```python
from build123d import *

# Parameters (mm, degrees)
F0_R     = 20
F0_R_2   = 2.25
F1_DEPTH = 22
F2_R     = 20
F2_R_2   = 14.25
F3_DEPTH = 7
F5_DEPTH = 13


with BuildPart() as f1:
    # F0 (on Right) → F1 (new body)
    with BuildSketch(Plane.YZ):
        Circle(F0_R)
        with Locations((-9.526279, -5.5)):
            Circle(F0_R_2, mode=Mode.SUBTRACT)
        with Locations((9.526279, -5.5)):
            Circle(F0_R_2, mode=Mode.SUBTRACT)
        with Locations((0, 11)):
            Circle(F0_R_2, mode=Mode.SUBTRACT)
    extrude(amount=F1_DEPTH)

    # F2 (on face) → F3 (join)
    with BuildSketch(Plane(origin=(0, 0, 0), x_dir=(0, -1, 0), z_dir=(-1, 0, 0))):
        Circle(F2_R)
        Circle(F2_R_2, mode=Mode.SUBTRACT)
    extrude(amount=F3_DEPTH)

    # F4 (on face) → F5 (cut)
    with BuildSketch(Plane.YZ.offset(22)):
        Polygon((3.752777, 6.5), (-3.752777, 6.5), (-7.505553, 0), (-3.752777, -6.5), (3.752777, -6.5), (7.505553, 0), align=None)
    extrude(amount=-F5_DEPTH, mode=Mode.SUBTRACT)


solid = f1.part
```
Input: part model. Units: mm. Frame: model coordinates. A direction names the side the tool comes from. Round coordinates to 2 decimals unless told otherwise and drop trailing zeros. Loops run counter-clockwise (first coordinate to the right, second up) from the corner with the lowest first, then second, coordinate; pieces in that order, holes last. Notation, with made-up numbers: M 8,-36.5 L 39,-36.5 A22 cw 39,-2.5 Z; hole C 27,3.5 d7. An arc over 180 degrees is marked long. Answer in a Markdown table with one row per item. Add a question column.
1. Section C-C (x = 5). Output: boundary loops of the cut face in (y, z), and give its area (3 significant figures).
2. Set-up query: faces 1 (the face through (-3.451, -13.163, -5.458)), 2 (the face through (10.85, -0.29, 13.23)), 3 (the face through (16, 0, 6.5)). Return all of +Z, -Z, +X, -X, +Y, -Y with unobstructed straight access to the full face (end or side cutting, diameter ignored); none if empty.
3. Contact query for flat-ended pins moving along their axis: pin 1 (4 mm diameter, centred on y = -9.53, z = -5.5, fed in from -X); pin 2 (10 mm diameter, centred on x = 16.5, z = -7.5, fed in from -Y); pin 3 (1 mm diameter, centred on x = 5.5, y = -5, fed in from -Z); pin 4 (4 mm diameter, centred on x = 17.5, y = -1.5, fed in from +Z). Output: stop coordinate, or through.
4. Section D-D (z = -9.5). Output: boundary loops of the cut face in (x, y).
5. Mould query, pull axis Z, two halves, no side actions, for faces 4 (the face through (10.85, -7.38, -4.82)), 5 (the face through (-7, 5, 14)), 6 (the face through (15.59, -5.66, -3.2)). Classes: released by +Z, released by -Z, zero draft, split by the parting line, or undercut.
6. Section B-B (z = 11). Output: boundary loops of the cut face in (x, y).
7. Section A-A (y = 0). Output: boundary loops of the cut face in (x, z), and give its area (4 significant figures).
8. Ray query, probe 1 along Z at (x, y) = (17, 0); probe 2 along Y at (x, z) = (18.25, -7) (3 decimals); probe 3 along Y at (x, z) = (12.5, 0). Return the intervals inside material, ascending.
Values follow:
| question | item | result |
|---|---|---|
| 1 | outline | C 0,0 d40; hole C -9.53,-5.5 d4.5; hole C 0,11 d4.5; hole C 9.53,-5.5 d4.5 |
| 1 | area | 1,210 mm^2 |
| 2 | face 1 | -X |
| 2 | face 2 | +X, -X |
| 2 | face 3 | +X |
| 3 | pin 1 | through |
| 3 | pin 2 | y = -19.84 |
| 3 | pin 3 | z = -19.49 |
| 3 | pin 4 | z = 20 |
| 4 | outline | M -7,-17.6 L 22,-17.6 L 22,17.6 L -7,17.6 L -7,10.62 L 0,10.62 L 0,-10.62 L -7,-10.62 Z |
| 5 | face 4 | undercut |
| 5 | face 5 | zero draft |
| 5 | face 6 | undercut |
| 6 | outline | M -7,-16.7 L 22,-16.7 L 22,-2.25 L 0,-2.25 L 0,-9.06 L -7,-9.06 Z; M -7,9.06 L 0,9.06 L 0,2.25 L 22,2.25 L 22,16.7 L -7,16.7 Z |
| 7 | outline | M -7,-20 L 22,-20 L 22,-6.5 L 9,-6.5 L 9,6.5 L 22,6.5 L 22,8.75 L 0,8.75 L 0,-14.25 L -7,-14.25 Z; M -7,14.25 L 0,14.25 L 0,13.25 L 22,13.25 L 22,20 L -7,20 Z |
| 7 | area | 692.5 mm^2 |
| 8 | probe 1 | -20 to -6.5, 6.5 to 8.75, 13.25 to 20 |
| 8 | probe 2 | -18.735 to -11.203, -7.849 to 7.849, 11.203 to 18.735 |
| 8 | probe 3 | -20 to -7.51, 7.51 to 20 |
